Here's how the part is built. I have some questions about the finished solid (model axes, mm). A direction names the side the tool comes from. Give positions to 0.01 mm unless a question says otherwise; leave off trailing zeros. Order: outer loops, then holes, each group sorted by start corner. A loop starts at its lowest first (then second) coordinate and runs counter-clockwise, first axis right, second up.
Autodesk Inventor part; units mm, degrees
ref_plane "YZ Plane" through (0, 0, 0) normal (1, 0, 0) x (0, 1, 0)
ref_plane "XZ Plane" through (0, 0, 0) normal (0, 1, 0) x (-1, 0, 0)
ref_plane "XY Plane" through (0, 0, 0) normal (0, 0, 1) x (1, 0, 0)
sketch "Sketch1" plane through (0, 0, 0) normal (0, 1, 0) x (-1, 0, 0)
  line L0 (6.225, -11.4) -> (-6.225, -11.4)
  line L1 (-6.225, -11.4) -> (-6.225, 11.4)
  line L2 (-6.225, 11.4) -> (6.225, 11.4)
  line L3 (6.225, 11.4) -> (6.225, -11.4)
  line L4 (0, 0) -> (0, -6.7915)
  line L5 (0, 0) -> (-3.4264, 0)
  point P0 (0, -11.4)
  point P1 (-6.225, 0)
  dimension "d0" = 12.45
  dimension "d1" = 22.8
extrude "Extrusion1" add sketch "Sketch1" along normal blind 16
sketch "Sketch2" plane through (0, 16, 0) normal (0, 1, 0) x (1, 0, 0)
  line L0 (-6.225, 11.4) -> (-6.225, -11.4)
  line L1 (6.225, -11.4) -> (6.225, 11.4)
  line L2 (6.225, -16.115) -> (-6.225, -16.115)
  line L3 (-6.225, -16.115) -> (-6.225, 16.115)
  line L4 (-6.225, 16.115) -> (6.225, 16.115)
  line L5 (6.225, 16.115) -> (6.225, -16.115)
  point P0 (0, 0)
  point P1 (-6.225, 0)
  point P2 (6.225, 0)
  dimension "d4" = 32.23
extrude "Extrusion2" add sketch "Sketch2" along normal blind 2
sketch "Sketch3" plane through (0, 18, 0) normal (0, 1, 0) x (1, 0, 0)
  line L0 (-6.225, 11.4) -> (6.225, 11.4)
  line L1 (6.225, 11.4) -> (6.225, -11.4)
  line L2 (6.225, -11.4) -> (-6.225, -11.4)
  line L3 (-6.225, -11.4) -> (-6.225, 11.4)
  line L4 (6.225, -16.115) -> (-6.225, -16.115)
  line L5 (-6.225, -16.115) -> (-6.225, 16.115)
  line L6 (-6.225, 16.115) -> (6.225, 16.115)
  line L7 (6.225, 16.115) -> (6.225, -16.115)
  line L8 (6.225, -16.115) -> (-6.225, -16.115)
  line L9 (-6.225, -16.115) -> (-6.225, 16.115)
  line L10 (-6.225, 16.115) -> (6.225, 16.115)
  line L11 (6.225, 16.115) -> (6.225, -16.115)
  point P0 (0, 0)
extrude "Extrusion3" add sketch "Sketch3" along normal blind 4 contours L0 L1 L2 L3
sketch "Sketch4" plane through (0, 22, 0) normal (0, 1, 0) x (1, 0, 0)
  line L0 (-6.225, 11.4) -> (-6.225, -11.4)
  line L1 (6.225, -11.4) -> (6.225, 11.4)
  circle A0 centre (0, 0) radius 6.225
  circle A1 centre (0, 0) radius 1.5
  point P0 (0, 0)
  dimension "d10" = 3
extrude "Extrusion4" add sketch "Sketch4" along normal blind 4 contours A0 | A1
sketch "Sketch5" plane through (0, 18, 0) normal (0, 1, 0) x (1, 0, 0)
  line L0 (-6.225, -16.115) -> (6.225, -16.115)
  line L1 (6.225, -16.115) -> (6.225, -11.4)
  circle A0 centre (0, -14.615) radius 1
  line L2 (0.5, -16.115) -> (-0.5, -16.115)
  line L3 (-0.5, -16.115) -> (-0.5, -15.115)
  line L4 (-0.5, -15.115) -> (0.5, -15.115)
  line L5 (0.5, -15.115) -> (0.5, -16.115)
  point P0 (0, 0)
  point P1 (0, -16.115)
  dimension "d15" = 2
  dimension "d16" = 1.5
  dimension "d17" = 1
  dimension "d18" = 1
  dimension "d19" = 6.225
extrude "Extrusion5" cut sketch "Sketch5" against normal blind 4
mirror "Mirror3" about plane through (0, 0, 0) normal (0, 0, 1) of "Extrusion5"
sketch "Sketch11" plane through (0, 26, 0) normal (0, 1, 0) x (1, 0, 0)
  arc A0 (6.225, 0) -> (6.225, 0) centre (0, 0) ccw
  circle A1 centre (0, 0) radius 2.5
  point P0 (0, 0)
  dimension "d49" = 5
extrude "Extrusion11" add sketch "Sketch11" along normal blind 2 contours A1
properties material "PPS Plastic"
Q1. If we section it at C-C on z = 3.5: List the corners of the cut face in (x, y) for me (3 decimals), plus the area to 3 significant figures.
Filled sheet:
outline: (-6.225, 0) - (6.225, 0) - (6.225, 22) - (5.148, 22) - (5.148, 26) - (-5.148, 26) - (-5.148, 22) - (-6.225, 22) - close
area: 315 mm2
Q2. I'm going to push flat-ended pins straight in: P1, Ø1.2, axis at x = -1, y = 20, coming from the +Z side; P2, Ø1.2, axis at x = 2.5, y = 20, coming from the -Z side; P3, Ø1, axis at x = -0.5, z = 12.5, coming from the -Y side. Where does each tip first touch, or does it pass through?
Filled sheet:
P1: stops at z = 11.4
P2: stops at z = -11.4
P3: stops at y = 16
Q3. I need wall thicknesses on L1, parallel to Z at x = 0, y = 17.1 (3 decimals); L2, parallel to Y at x = -2, z = 4.5; L3, parallel to Z at x = 3.75, y = 21.5. Which ranges of each line are inside material? Lowest first, please.
Filled sheet:
L1: z = -13.615 to 13.615
L2: y = 0 to 26
L3: z = -11.4 to 11.4
Q4. If we section it at B-B on x = 0: List the corners of the cut face in (y, z) for me (3 decimals).
Filled sheet:
outline: (0, -11.4) - (16, -11.4) - (16, -13.615) - (18, -13.615) - (18, -11.4) - (22, -11.4) - (22, -6.225) - (26, -6.225) - (26, -2.5) - (28, -2.5) - (28, 2.5) - (26, 2.5) - (26, 6.225) - (22, 6.225) - (22, 11.4) - (18, 11.4) - (18, 13.615) - (16, 13.615) - (16, 11.4) - (0, 11.4) - close
Q5. If we section it at A-A on z = 14: List the corners of the cut face in (x, y) for me (3 decimals).
Filled sheet:
outline: (-6.225, 16) - (-0.789, 16) - (-0.789, 18) - (-6.225, 18) - close; (0.789, 16) - (6.225, 16) - (6.225, 18) - (0.789, 18) - close
Q6. For faces 1 (the face through (0, 20, 11.4)), 2 (the face through (0, 8, 11.4)), 3 (the face through (0, 18, -13)), 4 (the face through (-4.588, 23.972, 4.207)), 5 (the face through (0, 16, -13)), which set-ups out of +Z, -Z, +X, -X, +Y, -Y let a thin tool reach every point of the face, with its end or its side?
Filled sheet:
face 1: +Z, +X, -X, +Y
face 2: +Z, +X, -X, -Y
face 3: -Z, +X, -X, +Y
face 4: +Y
face 5: -Z, +X, -X, -Y
Q7. If we section it at D-D on y = 5.5: List the corners of the cut face in (x, z) for me (3 decimals).
Filled sheet:
outline: (-6.225, -11.4) - (6.225, -11.4) - (6.225, 11.4) - (-6.225, 11.4) - close
